Here's how the part is built. I have some questions about the finished solid (model axes, mm). A direction names the side the tool comes from. Give positions to 0.01 mm unless a question says otherwise; leave off trailing zeros. Loops run counter-clockwise (first coordinate to the right, second up) from the corner with the lowest first, then second, coordinate; pieces in that order, holes last.
Q1. If we section it at A-A (z = -21.5): Please give me the cut outline in (x, y), plus the area to 3 significant figures.
Q2. I need wall thicknesses on line 1 (Z direction, x = -25, y = 1.3); line 2 (Z direction, x = 26, y = 2); line 3 (X direction, y = 3.1, z = 10). Which ranges of each line are inside material? Lowest first, please.
Q3. Will these pins go through, and if not, where does the flat tip stop? P1, Ø0.6, axis at x = 27, y = 3.5, coming from the -Z side; P2, Ø1.6, axis at x = 27, y = 4.5, coming from the +Z side; P3, Ø6.5, axis at x = -6.5, z = 10, coming from the +Y side.
Q4. For faces 4 (the face through (27, 3, 12.45)), 5 (the face through (-5.53, 3.29, -5.37)), which set-ups out of +Z, -Z, +X, -X, +Y, -Y let a thin tool reach every point of the face, with its end or its side?
Q5. We'd pull the mould along X, two halves only. Please class faces 1 (the face through (32.15, 2.96, -21.99)), 2 (the face through (30.55, 2.96, -14.94)), 3 (the face through (-32.15, 2.96, 21.99)): +X half, -X half, draft (parallel to the pull), parting line (faces both ways), or undercut.
from build123d import *

# Parameters (mm, degrees)
EXTRUDE_1_DEPTH             = 6
SKETCH_2_R                  = 2.55
CUT_EXTRUDE_1_DEPTH         = 7
CUT_EXTRUDE_2_DEPTH         = 7
HOLE_WIZARD_M52_D           = 5.5
HOLE_WIZARD_M52_CSINK_D     = 11.2
HOLE_WIZARD_M52_CSINK_ANGLE = 90
HOLE_WIZARD_M51_D           = 5.5
HOLE_WIZARD_M51_CSINK_D     = 11.2
HOLE_WIZARD_M51_CSINK_ANGLE = 90


with BuildPart() as part:
    # Эскиз1 → Бобышка-Вытянуть1 (new body)
    with BuildSketch(Plane(origin=(0, 0, 0), x_dir=(1, 0, 0), z_dir=(0, 1, 0))):
        with BuildLine():
            Line((-25, -25), (25, -25))
            ThreePointArc((25, -25), (32.071067812, -22.071067812), (35, -15))
            Line((35, -15), (35, 15))
            ThreePointArc((35, 15), (32.071067812, 22.071067812), (25, 25))
            Line((25, 25), (-25, 25))
            ThreePointArc((-25, 25), (-32.071067812, 22.071067812), (-35, 15))
            Line((-35, 15), (-35, -15))
            ThreePointArc((-35, -15), (-32.071067812, -22.071067812), (-25, -25))
        make_face()
    extrude(amount=EXTRUDE_1_DEPTH)

    # Эскиз2 → Вырез-Вытянуть1 (cut, through all)
    with BuildSketch(Plane.XZ):
        with Locations((-25, -15)):
            Circle(SKETCH_2_R)
        with Locations((-25, 15)):
            Circle(SKETCH_2_R)
        with BuildLine():
            Line((28, -17.55), (26, -17.55))
            ThreePointArc((26, -17.55), (23.45, -15), (26, -12.45))
            Line((26, -12.45), (28, -12.45))
            ThreePointArc((28, -12.45), (30.55, -15), (28, -17.55))
        make_face()
        with BuildLine():
            Line((28, 17.55), (26, 17.55))
            ThreePointArc((26, 17.55), (23.45, 15), (26, 12.45))
            Line((26, 12.45), (28, 12.45))
            ThreePointArc((28, 12.45), (30.55, 15), (28, 17.55))
        make_face()
    extrude(amount=-CUT_EXTRUDE_1_DEPTH, mode=Mode.SUBTRACT)

    # Эскиз3 → Вырез-Вытянуть2 (cut, through all)
    with BuildSketch(Plane.XZ):
        with BuildLine():
            Line((-35, -2), (-35, 2))
            ThreePointArc((-35, 2), (-34.414213562, 0.585786438), (-33, 0))
            ThreePointArc((-33, 0), (-34.414213562, -0.585786438), (-35, -2))
        make_face()
    extrude(amount=-CUT_EXTRUDE_2_DEPTH, mode=Mode.SUBTRACT)

    # Зенковка для  винта с потайной головкой с внутренним шестигранником M52 (through all)
    with Locations(Plane(origin=(0, 6, 0), x_dir=(1, 0, 0), z_dir=(0, 1, 0))):
        with Locations((-6.159381211, -9.040339254), (-6.159381211, 8.192585184)):
            CounterSinkHole(HOLE_WIZARD_M52_D / 2, HOLE_WIZARD_M52_CSINK_D / 2, counter_sink_angle=HOLE_WIZARD_M52_CSINK_ANGLE)

    # Зенковка для  винта с потайной головкой с внутренним шестигранником M51 (through all)
    with Locations(Plane(origin=(0, 0, 0), x_dir=(-1, 0, 0), z_dir=(0, -1, 0))):
        with Locations((6.5, -10), (6.5, 10)):
            CounterSinkHole(HOLE_WIZARD_M51_D / 2, HOLE_WIZARD_M51_CSINK_D / 2, counter_sink_angle=HOLE_WIZARD_M51_CSINK_ANGLE)


solid = part.part
Check sheet entries:
1. outline: (-32.6, 0) - (32.6, 0) - (32.6, 6) - (-32.6, 6) - close
1. area: 391 mm2
2. line 1: z = -25 to -17.55, -12.45 to 12.45, 17.55 to 25
2. line 2: z = -24.95 to -17.55, -12.45 to 12.45, 17.55 to 24.95
2. line 3: x = -35 to -9.25, -3.58 to 35
3. P1: stops at z = -24.85
3. P2: stops at z = 24.93
3. P3: stops at y = 4.67
4. face 4: +Y, -Y
4. face 5: +Y
5. face 1: +X half
5. face 2: undercut
5. face 3: -X half
